Could you check a few things on this model? Use its own coordinates, in mm. A direction names the side the tool comes from. Coordinates: 2 decimals unless noted, no trailing zeros. Write each loop counter-clockwise with the first axis right and the second up, starting at its lowest first coordinate (ties: lowest second). Pieces come first, ordered by that corner, then holes.
```python
from build123d import *

# Parameters (mm, degrees)
SKETCH1_R           = 55
BOSS_EXTRUDE1_DEPTH = 5
SKETCH2_W           = 30
SKETCH2_H           = 14
BOSS_EXTRUDE2_DEPTH = 30
SKETCH6_R           = 2.05
CUT_EXTRUDE3_DEPTH  = 30
SKETCH7_W           = 30
SKETCH7_H           = 3.4
CUT_EXTRUDE4_DEPTH  = 6
SKETCH10_R          = 1.6
CUT_EXTRUDE5_DEPTH  = 6
SKETCH11_W          = 30
SKETCH11_H          = 17.3
CUT_EXTRUDE6_DEPTH  = 1.5
BOSS_EXTRUDE5_DEPTH = 5
SKETCH16_R          = 4
BOSS_EXTRUDE6_DEPTH = 5
SKETCH17_R          = 1.6
CUT_EXTRUDE8_DEPTH  = 97.306801421
SKETCH13_R          = 5
CUT_EXTRUDE9_DEPTH  = 2
CIRPATTERN3_COUNT   = 4


with BuildPart() as part:
    # Sketch1 → Boss-Extrude1 (new body)
    with BuildSketch(Plane(origin=(0, 0, 0), x_dir=(1, 0, 0), z_dir=(0, 1, 0))):
        with Locations(Location((0, 0, 0), (0, 0, 270))):
            Circle(SKETCH1_R)
    extrude(amount=BOSS_EXTRUDE1_DEPTH)

    # Sketch2 → Boss-Extrude2 (add)
    with BuildSketch(Plane(origin=(0, 5, 0), x_dir=(1, 0, 0), z_dir=(0, 1, 0))):
        with Locations((0, -27.9)):
            Rectangle(SKETCH2_W, SKETCH2_H)
    extrude(amount=BOSS_EXTRUDE2_DEPTH)

    # Sketch6 → Cut-Extrude3 (cut)
    with BuildSketch(Plane(origin=(0, 35, 0), x_dir=(1, 0, 0), z_dir=(0, 1, 0))):
        with Locations(Location((-6, -24, 0), (0, 0, 270))):
            Circle(SKETCH6_R)
        with Locations(Location((0, -24, 0), (0, 0, 270))):
            Circle(SKETCH6_R)
        with Locations(Location((6, -24, 0), (0, 0, 270))):
            Circle(SKETCH6_R)
    extrude(amount=-CUT_EXTRUDE3_DEPTH, mode=Mode.SUBTRACT)

    # Sketch7 → Cut-Extrude4 (cut)
    with BuildSketch(Plane(origin=(0, 0, 20.9), x_dir=(-1, 0, 0), z_dir=(0, 0, -1))):
        with Locations((0, 6.7)):
            Rectangle(SKETCH7_W, SKETCH7_H)
        with Locations((0, 27.4)):
            Rectangle(SKETCH7_W, SKETCH7_H)
    extrude(amount=-CUT_EXTRUDE4_DEPTH, mode=Mode.SUBTRACT)

    # Sketch10 → Cut-Extrude5 (cut)
    with BuildSketch(Plane.XZ):
        with Locations(Location((-28.284271247, 28.284271247, 0), (0, 0, 270))):
            Circle(SKETCH10_R)
        with Locations(Location((28.284271247, 28.284271247, 0), (0, 0, 270))):
            Circle(SKETCH10_R)
        with Locations(Location((28.284271247, -28.284271247, 0), (0, 0, 270))):
            Circle(SKETCH10_R)
        with Locations(Location((-28.284271247, -28.284271247, 0), (0, 0, 270))):
            Circle(SKETCH10_R)
    extrude(amount=-CUT_EXTRUDE5_DEPTH, mode=Mode.SUBTRACT)

    # Sketch11 → Cut-Extrude6 (cut)
    with BuildSketch(Plane(origin=(0, 0, 20.9), x_dir=(-1, 0, 0), z_dir=(0, 0, -1))):
        with Locations((0, 17.05)):
            Rectangle(SKETCH11_W, SKETCH11_H)
    extrude(amount=-CUT_EXTRUDE6_DEPTH, mode=Mode.SUBTRACT)

    # Sketch14 → Boss-Extrude5 (add)
    with BuildSketch(Plane.XZ):
        Polygon((-26, -48.466483264), (-26, -75), (26, -75), (26, -25), (-26, -25), align=None)
    extrude(amount=-BOSS_EXTRUDE5_DEPTH)

    # Sketch16 → Boss-Extrude6 (add)
    with BuildSketch(Plane(origin=(0, 5, 0), x_dir=(1, 0, 0), z_dir=(0, 1, 0))):
        with Locations(Location((-21, 68, 0), (0, 0, 270))):
            Circle(SKETCH16_R)
        with Locations(Location((21.07, 68, 0), (0, 0, 270))):
            Circle(SKETCH16_R)
        with Locations(Location((-21, 19.96, 0), (0, 0, 270))):
            Circle(SKETCH16_R)
        with Locations(Location((21.07, 19.96, 0), (0, 0, 270))):
            Circle(SKETCH16_R)
    extrude(amount=BOSS_EXTRUDE6_DEPTH)

    # Sketch17 → Cut-Extrude8 (cut, through all)
    with BuildSketch(Plane(origin=(0, 10, 0), x_dir=(1, 0, 0), z_dir=(0, 1, 0))):
        with Locations(Location((-21, 68, 0), (0, 0, 270))):
            Circle(SKETCH17_R)
        with Locations(Location((21.07, 68, 0), (0, 0, 270))):
            Circle(SKETCH17_R)
        with Locations(Location((21.07, 19.96, 0), (0, 0, 270))):
            Circle(SKETCH17_R)
        with Locations(Location((-21, 19.96, 0), (0, 0, 270))):
            Circle(SKETCH17_R)
    extrude(amount=-CUT_EXTRUDE8_DEPTH, mode=Mode.SUBTRACT)

    # Sketch13 → Cut-Extrude9 (cut)
    with BuildSketch(Plane(origin=(0, 5, 0), x_dir=(1, 0, 0), z_dir=(0, 1, 0))):
        with Locations(Location((-28.284271247, 28.284271247, 0), (0, 0, 270))):
            Circle(SKETCH13_R)
    cut_extrude9 = extrude(amount=-CUT_EXTRUDE9_DEPTH, mode=Mode.SUBTRACT)

    # CirPattern3: Cut-Extrude9 ×4 about axis
    cirpattern3_axis = Axis((0, 0, 0), (0, 1, 0))
    for i in range(1, CIRPATTERN3_COUNT):
        add(cut_extrude9.rotate(cirpattern3_axis, i * 360 / CIRPATTERN3_COUNT), mode=Mode.SUBTRACT)


solid = part.part
```
1. I want a section at B-B on x = 21.07. Please give me the cut outline in (y, z).
Verdict:
outline: (0, -75) - (5, -75) - (5, -72) - (10, -72) - (10, -69.6) - (0, -69.6) - close; (0, -66.4) - (10, -66.4) - (10, -64) - (5, -64) - (5, -23.96) - (10, -23.96) - (10, -21.56) - (0, -21.56) - close; (0, -18.36) - (10, -18.36) - (10, -15.96) - (5, -15.96) - (5, 50.8) - (0, 50.8) - close
2. For pin 1 (1.7 mm diameter, centred on x = 5, y = 7.5, fed in from -Z); pin 2 (8 mm diameter, centred on x = 30.5, z = 28, fed in from +Y); pin 3 (4 mm diameter, centred on x = -20.5, z = -20.5, fed in from +Y), each with a flat end and sliding along its axis, tell me the tip position at first contact or that it passes through.
Verdict:
pin 1: stops at z = 26.9
pin 2: stops at y = 5
pin 3: stops at y = 10
3. Please list where these lines run through material, in increasing order: line 1 along X through (y, z) = (21, 24); line 2 along X through (y, z) = (3, -68); line 3 along X through (y, z) = (5.5, -19.96).
Verdict:
line 1: x = -15 to -8.05, -3.95 to -2.05, 2.05 to 3.95, 8.05 to 15
line 2: x = -26 to -22.6, -19.4 to 19.47, 22.67 to 26
line 3: x = -25 to -22.6, -19.4 to -17, 17.07 to 19.47, 22.67 to 25.07
4. On a 3-axis mill with a long thin cutter (end or side, diameter ignored), from which of +Z, -Z, +X, -X, +Y, -Y can I reach the whole of each face in a straight line? I mean faces 1 (the face through (-26, 2, -62)), 2 (the face through (15, 20, 30)), 3 (the face through (-11, 17, 22.4)), 4 (the face through (-17, 7, -20)). Say none if no direction works.
Verdict:
face 1: -Z, -X, +Y, -Y
face 2: +Z, -Z, +X, +Y
face 3: -Z, +X, -X
face 4: +Y
5. If we mould it in two halves opening along Y, with no side actions, what happens to faces 5 (the face through (-1, 0, -9)), 6 (the face through (0, 32, 20.9)), 7 (the face through (0.2, 25.7, 26.6))? For each: pulls with the +Y half, pulls with the -Y half, needs draft (parallel to the pull), parting line crosses it, or undercut.
Verdict:
face 5: pulls with the -Y half
face 6: needs draft
face 7: undercut
6. I want a section at C-C on y = 20. Please give me the cut outline in (x, z).
Verdict:
outline: (-15, 22.4) - (-7.28, 22.4) arc R2.05 cw (long way) to (-4.72, 22.4) - (-1.28, 22.4) arc R2.05 cw (long way) to (1.28, 22.4) - (4.72, 22.4) arc R2.05 cw (long way) to (7.28, 22.4) - (15, 22.4) - (15, 34.9) - (-15, 34.9) - close
7. I want a section at A-A on z = -19.96. Please give me the cut outline in (x, y), plus the area to 3 significant figures.
Verdict:
outline: (-51.25, 0) - (-22.6, 0) - (-22.6, 10) - (-25, 10) - (-25, 5) - (-51.25, 5) - close; (-19.4, 0) - (19.47, 0) - (19.47, 10) - (17.07, 10) - (17.07, 5) - (-17, 5) - (-17, 10) - (-19.4, 10) - close; (22.67, 0) - (51.25, 0) - (51.25, 5) - (25.07, 5) - (25.07, 10) - (22.67, 10) - close
area: 529 mm2
8. I want a section at D-D on z = 0. Please give me the cut outline in (x, y), plus the area to 3 significant figures.
Verdict:
outline: (-55, 0) - (55, 0) - (55, 5) - (-55, 5) - close
area: 550 mm2
